from build123d import *

# Parameters (mm, degrees)
F0_W      = 20
F0_H      = 20
F0_W_2    = 18.4
F0_H_2    = 18.4
F1_DEPTH  = 2
F2_DEPTH  = 2.5
F4_DEPTH  = 2
F5_SIZE2  = 0.334
F5_SIZE   = 0.167
F6_R      = 4
F7_DEPTH  = 4.501
F8_SIZE2  = 0.334
F8_SIZE   = 0.167
F9_SIZE2  = 0.334
F9_SIZE   = 0.167
F10_W     = 3
F10_H     = 1.2
F11_DEPTH = 2.167
F12_R     = 3
F13_DEPTH = 6


with BuildPart() as f1:
    # F0 (on Top) → F1 (new body)
    with BuildSketch(Plane.XY):
        with Locations((3.0281848833, -2.0047442615)):
            Rectangle(F0_W, F0_H)
        with Locations((3.0281848833, -2.0047442615)):
            Rectangle(F0_W_2, F0_H_2, mode=Mode.SUBTRACT)
        with Locations((3.0281848833, -2.0047442615)):
            Rectangle(F0_W_2, F0_H_2)
    extrude(amount=-F1_DEPTH)

    # F0 (on Top) → F2 (join)
    with BuildSketch(Plane.XY):
        with Locations((3.0281848833, -2.0047442615)):
            Rectangle(F0_W, F0_H)
        with Locations((3.0281848833, -2.0047442615)):
            Rectangle(F0_W_2, F0_H_2, mode=Mode.SUBTRACT)
    extrude(amount=F2_DEPTH)

    # F3 (on face) → F4 (cut)
    with BuildSketch(Plane(origin=(0, 0, -2), x_dir=(1, 0, 0), z_dir=(0, 0, -1))):
        Polygon((4.5281848833, -5.9952557385), (3.0281848833, -5.9952557385), (1.5281848833, -5.9952557385), (1.5281848833, -7.9952557385), (4.5281848833, -7.9952557385), align=None)
    extrude(amount=-F4_DEPTH, mode=Mode.SUBTRACT)

    # F5
    f5_edges = [f1.edges().sort_by_distance(p)[0] for p in [
        (13.028185, -2.004744, -2),
        (3.028185, -12.004744, -2),
        (-6.971815, -2.004744, -2),
        (-2.721815, 7.995256, -2),
        (1.528185, 6.995256, -2),
        (3.028185, 5.995256, -2),
        (4.528185, 6.995256, -2),
        (8.778185, 7.995256, -2),
    ]]
    f5_side = f1.faces().sort_by_distance((3.028185, -2.1418, -2))[0]
    chamfer(f5_edges, length=F5_SIZE, length2=F5_SIZE2, reference=f5_side)

    # F6 (on face) → F7 (cut, through all)
    with BuildSketch(Plane(origin=(0, 0, -2), x_dir=(1, 0, 0), z_dir=(0, 0, -1))):
        with Locations((3.0281848833, 2.0047442615)):
            Circle(F6_R)
    extrude(amount=-F7_DEPTH, mode=Mode.SUBTRACT)

    # F8
    f8_edges = [f1.edges().sort_by_distance(p)[0] for p in [
        (-0.971815, -2.004744, -2),
        (-0.971815, -2.004744, 0),
    ]]
    chamfer(f8_edges, length=F8_SIZE, length2=F8_SIZE2)

    # F9
    f9_edges = [f1.edges().sort_by_distance(p)[0] for p in [
        (3.028185, 7.995256, 2.5),
        (-6.971815, -2.004744, 2.5),
        (3.028185, -12.004744, 2.5),
        (13.028185, -2.004744, 2.5),
        (-6.171815, -2.004744, 2.5),
        (3.028185, 7.195256, 2.5),
        (12.228185, -2.004744, 2.5),
        (3.028185, -11.204744, 2.5),
    ]]
    f9_side = f1.faces().sort_by_distance((3.028185, 7.712413, 2.5))[0]
    chamfer(f9_edges, length=F9_SIZE, length2=F9_SIZE2, reference=f9_side)

    # F10 (on face) → F11 (join)
    with BuildSketch(Plane.XY):
        Polygon((4.5281848833, 5.9952557385), (1.5281848833, 5.9952557385), (1.5281848833, 7.1952557385), (0.3281848833, 7.1952557385), (0.3281848833, 4.7952557385), (5.7281848833, 4.7952557385), (5.7281848833, 7.1952557385), (4.5281848833, 7.1952557385), align=None)
        with Locations((3.0281848833, 6.5952557385)):
            Rectangle(F10_W, F10_H)
    extrude(amount=F11_DEPTH)

    # F12 (on face) → F13 (join)
    with BuildSketch(Plane.XY):
        with Locations((-2.6718151167, -7.7047442615)):
            Circle(F12_R)
    extrude(amount=F13_DEPTH)


solid = f1.part
For this review, take the finished solid that the model builds, in its own axes (mm). A direction names the side the tool comes from. Give positions to 0.01 mm unless a question says otherwise; leave off trailing zeros. Loops run counter-clockwise (first coordinate to the right, second up) from the corner with the lowest first, then second, coordinate; pieces in that order, holes last.
Item 1: For line 1 along X through (y, z) = (5, 1.25); line 2 along Y through (x, z) = (12, 1.25); line 3 along X through (y, z) = (4.25, 0.5), list the stretches that pass through material, from the lowest coordinate up.
Item 2: Draft analysis for pull direction X (two halves, no side actions). For faces 1 (the flat face through (-6.172, -2, 1)), 2 (the flat face through (2.9, 7.995, 0.2)), 3 (the flat face through (-6.972, -2, 0)), state which applies: +X half, -X half, draft (parallel to the pull), parting line (faces both ways), or undercut.
Item 3: Tool access review of faces 4 (the flat face through (1.528, 7, -1)), 5 (the flat face through (3, 6, 2.167)), 6 (the flat face through (-1.5, -1.9, -2)): name each direction out of +Z, -Z, +X, -X, +Y, -Y from which nothing blocks a thin tool from reaching the whole face with its end or side.
Item 4: Take a section at B-B, the plane y = -8.25. State the section outline as (x, z) points, and give its area (3 significant figures).
Item 5: Take a section at C-C, the plane z = 5. State the section outline as (x, y) points, and give its area (3 significant figures).
Item 6: Insertion check: pin 1 (3 mm diameter, centred on x = 0, y = -2, fed in from +Z); pin 2 (0.5 mm diameter, centred on x = 3, z = -1, fed in from +Y); pin 3 (1.2 mm diameter, centred on x = 2, y = 5.5, fed in from +Z). Each pin has a flat end and moves straight along its axis. Give the tip position at first contact, or say it passes through.
Item 7: Take a section at A-A, the plane x = 11. State the section outline as (y, z) points.
Calculated:
1. line 1: x = -6.97 to -6.17, 0.33 to 5.73, 12.23 to 13.03
1. line 2: y = -12 to -11.2, 7.2 to 8
1. line 3: x = -6.97 to -6.17, 12.23 to 13.03
2. face 1: undercut
2. face 2: draft
2. face 3: -X half
3. face 4: -Z, +Y
3. face 5: +Z
3. face 6: -Z, +X, -X, +Y, -Y
4. outline: (-6.97, -1.67) - (-6.8, -2) - (12.86, -2) - (13.03, -1.67) - (13.03, 2.17) - (12.86, 2.5) - (12.4, 2.5) - (12.23, 2.17) - (12.23, 0) - (0.28, 0) - (0.28, 6) - (-5.62, 6) - (-5.62, 0) - (-6.17, 0) - (-6.17, 2.17) - (-6.34, 2.5) - (-6.8, 2.5) - (-6.97, 2.17) - close
4. area: 79.2 mm2
5. outline: circle Ø6 at (-2.67, -7.7)
5. area: 28.3 mm2
6. pin 1: stops at z = 0
6. pin 2: stops at y = 6
6. pin 3: stops at z = 2.17
7. outline: (-12, -1.67) - (-11.84, -2) - (7.83, -2) - (8, -1.67) - (8, 2.17) - (7.83, 2.5) - (7.36, 2.5) - (7.2, 2.17) - (7.2, 0) - (-11.2, 0) - (-11.2, 2.17) - (-11.37, 2.5) - (-11.84, 2.5) - (-12, 2.17) - close
